Design review of the part built by this model. Coordinates are the model's own, in mm. Face numbers are marked on the shaded views. A direction names the side the tool comes from. Coordinates: 2 decimals unless noted, no trailing zeros. Write each loop counter-clockwise with the first axis right and the second up, starting at its lowest first coordinate (ties: lowest second). Pieces come first, ordered by that corner, then holes. Notation, with made-up numbers: (24.5, 85) - (67.5, 85) arc R10 cw to (67.5, 103) - close; hole circle Ø2 at (-15, 33). An arc over 180 degrees is marked (long way). Answer as CSV lines item,"result". Start each with the question number.
Q1. We need section D-D (z = 8). Write out the cut boundary in (x, y).
Q2. Mouldability with a two-part tool opening along X and no side actions: class the marked faces 1, 2 and 3 as pulls with the +X half, pulls with the -X half, needs draft (parallel to the pull), parting line crosses it, or undercut.
Q3. For line 1 along X through (y, z) = (4, -21); line 2 along X through (y, z) = (27.5, -2.5); line 3 along Z through (x, y) = (42, 22), list the stretches that pass through material, from the lowest coordinate up. Write a range as [from, to].
Q4. We need section C-C (y = 28.5). Write out the cut boundary in (x, z).
Q5. Machinability: for the marked faces 4 and 5, which of the approach directions +Z, -Z, +X, -X, +Y, -Y give a long, thin tool a straight path to every point of the face, cutting with its end or side? Answer none if there is none.
Q6. We need section A-A (z = -30.5). Write out the cut boundary in (x, y).
from build123d import *

# Parameters (mm, degrees)
SKETCH1_W           = 108.824103019
SKETCH1_H           = 66.04
BOSS_EXTRUDE4_DEPTH = 3.81
SKETCH5_W           = 108.824103019
SKETCH5_H           = 66.04
SKETCH5_W_2         = 93.0148
SKETCH5_H_2         = 60.9092
BOSS_EXTRUDE5_DEPTH = 12.7
SKETCH6_W           = 22.284444933
SKETCH6_H           = 10.320659342
CUT_EXTRUDE2_DEPTH  = 12.954
FILLET2_R           = 2.54
FILLET3_R           = 2.54
SKETCH8_W           = 9.964328511
SKETCH8_H           = 60.899089628
CUT_EXTRUDE4_DEPTH  = 8.128
SKETCH11_W          = 108.824103019
SKETCH11_H          = 66.04
SKETCH11_W_2        = 102.814143763
SKETCH11_H_2        = 60.899089628
BOSS_EXTRUDE6_DEPTH = 19.558


with BuildPart() as part:
    # Sketch1 → Boss-Extrude4 (new body)
    with BuildSketch(Plane(origin=(0, 0, 0), x_dir=(1, 0, 0), z_dir=(0, 1, 0))):
        with Locations((11.887002401, 13.227171797)):
            Rectangle(SKETCH1_W, SKETCH1_H)
    extrude(amount=BOSS_EXTRUDE4_DEPTH)

    # Sketch5 → Boss-Extrude5 (add)
    with BuildSketch(Plane(origin=(0, 3.81, 0), x_dir=(1, 0, 0), z_dir=(0, 1, 0))):
        with Locations((11.887002401, 13.227171797)):
            Rectangle(SKETCH5_W, SKETCH5_H)
        with Locations((16.771366144, 12.995675742)):
            Rectangle(SKETCH5_W_2, SKETCH5_H_2, mode=Mode.SUBTRACT)
    extrude(amount=BOSS_EXTRUDE5_DEPTH)

    # Sketch6 → Cut-Extrude2 (cut)
    with BuildSketch(Plane.ZY.offset(42.525049108)):
        with Locations((-32.297942904, 8.873970447)):
            Rectangle(SKETCH6_W, SKETCH6_H)
    extrude(amount=-CUT_EXTRUDE2_DEPTH, mode=Mode.SUBTRACT)

    # Fillet2
    fillet2_edges = [part.edges().sort_by_distance(p)[0] for p in [
        (11.887002402, 0, 19.792828203),
    ]]
    fillet(fillet2_edges, radius=FILLET2_R)

    # Fillet3
    fillet3_edges = [part.edges().sort_by_distance(p)[0] for p in [
        (11.887002402, 0, -46.247171797),
    ]]
    fillet(fillet3_edges, radius=FILLET3_R)

    # Sketch8 → Cut-Extrude4 (cut)
    with BuildSketch(Plane(origin=(0, 16.51, 0), x_dir=(1, 0, 0), z_dir=(0, 1, 0))):
        with Locations((-34.553213363, 12.990620556)):
            Rectangle(SKETCH8_W, SKETCH8_H)
    extrude(amount=-CUT_EXTRUDE4_DEPTH, mode=Mode.SUBTRACT)

    # Sketch11 → Boss-Extrude6 (add)
    with BuildSketch(Plane(origin=(0, 16.51, 0), x_dir=(1, 0, 0), z_dir=(0, 1, 0))):
        with Locations((11.887002401, 13.227171797)):
            Rectangle(SKETCH11_W, SKETCH11_H)
        with Locations((11.871694263, 12.990620556)):
            Rectangle(SKETCH11_W_2, SKETCH11_H_2, mode=Mode.SUBTRACT)
    extrude(amount=BOSS_EXTRUDE6_DEPTH)


solid = part.part
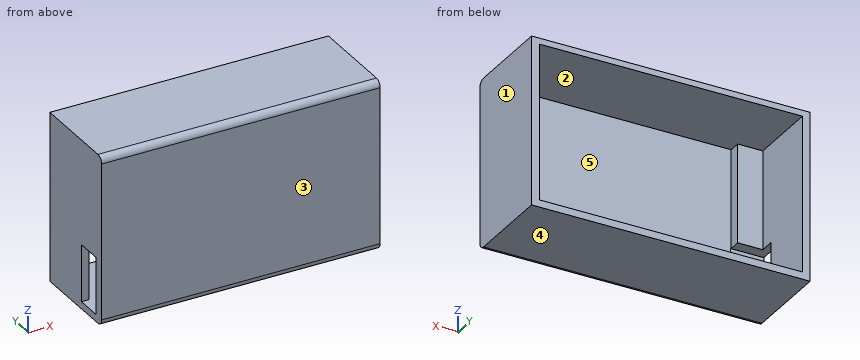
Results list:
1,outline,"(-42.53, 0) - (66.3, 0) - (66.3, 36.07) - (63.28, 36.07) - (63.28, 3.81) - (-29.74, 3.81) - (-29.74, 8.38) - (-39.54, 8.38) - (-39.54, 36.07) - (-42.53, 36.07) - close"
2,face 1,"pulls with the +X half"
2,face 2,"undercut"
2,face 3,"needs draft"
3,line 1,"x = [-42.53, -29.74], [63.28, 66.3]"
3,line 2,"x = [-42.53, -39.54], [63.28, 66.3]"
3,line 3,"z = [-46.25, -43.44], [17.46, 19.79]"
4,outline,"(-42.53, -46.25) - (66.3, -46.25) - (66.3, 19.79) - (-42.53, 19.79) - close; hole (-39.54, -43.44) - (63.28, -43.44) - (63.28, 17.46) - (-39.54, 17.46) - close"
5,face 4,"-Z, +X, -X, +Y, -Y"
5,face 5,"+Y"
6,outline,"(-42.53, 0) - (66.3, 0) - (66.3, 36.07) - (63.28, 36.07) - (63.28, 3.81) - (-29.57, 3.81) - (-29.57, 3.71) - (-42.53, 3.71) - close; (-42.53, 14.03) - (-39.54, 14.03) - (-39.54, 36.07) - (-42.53, 36.07) - close"
